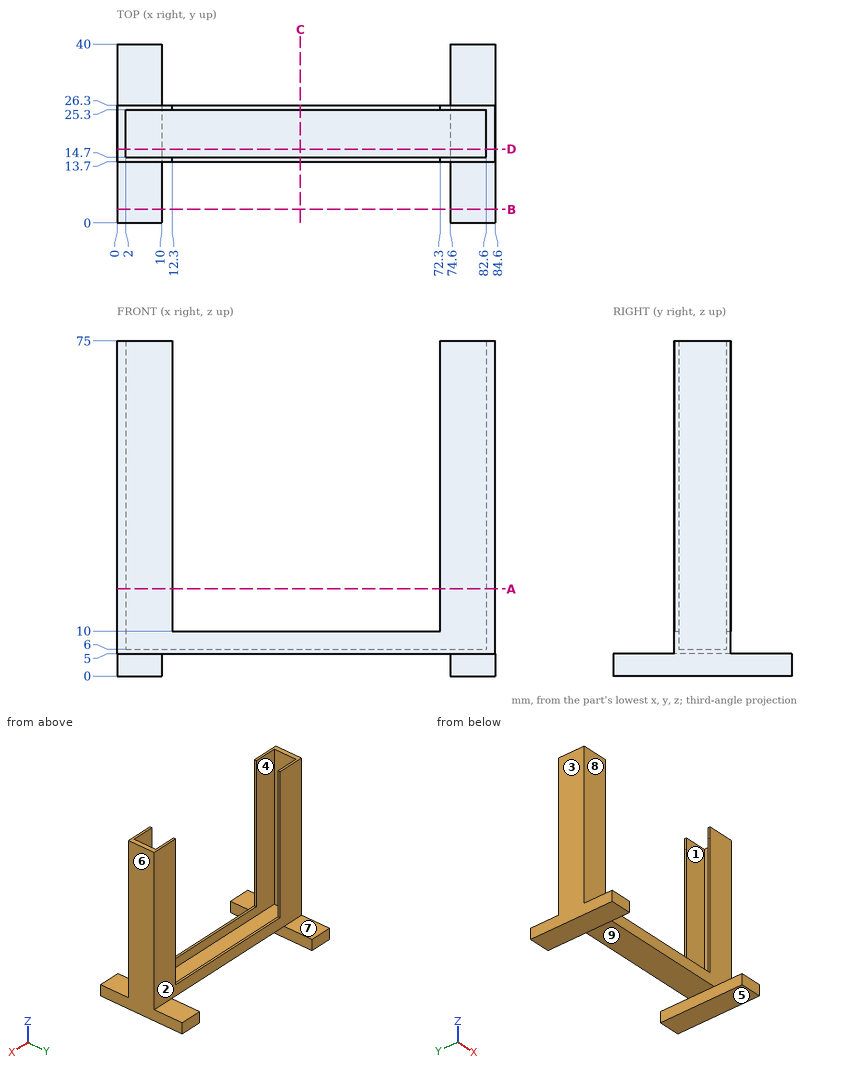
Could you check a few things on this drawing? It's one solid part, dimensions in mm from its lowest x, y, z. A direction names the side the tool comes from. Give positions to 0.01 mm unless a question says otherwise; leave off trailing zeros. Write each loop counter-clockwise with the first axis right and the second up, starting at its lowest first coordinate (ties: lowest second). Pieces come first, ordered by that corner, then holes. Notation, with made-up numbers: M -2.75,85 L 38.25,85 A8 cw 38.25,91 Z; hole C 8.25,-17 d8. An arc over 180 degrees is marked long. Put each result on its own line as item: value. Start each with the question number.
Item 1: Will these pins go through, and if not, where does the flat tip stop? pin 1 (5 mm diameter, centred on x = 3.5, y = 31.5, fed in from +Z); pin 2 (8.5 mm diameter, centred on x = 41.5, y = 22.5, fed in from +Z); pin 3 (6.5 mm diameter, centred on x = 37.5, y = 23, fed in from -Z).
Item 2: If we section it at B-B, the plane y = 3: Write out the boundary of the cut face in (x, z), then the cut area to 3 significant figures.
Item 3: Thinking about a two-plate mould opening in Y: for the marked faces 1, 2, 3 and 4, which applies, +Y half, -Y half, draft (parallel to the pull), parting line (faces both ways), or undercut?
Item 4: If we section it at C-C, the plane x = 41: Write out the boundary of the cut face in (y, z), then the cut area to 3 significant figures.
Item 5: If we section it at A-A, the plane z = 19.5: Write out the boundary of the cut face in (x, y), then the cut area to 3 significant figures.
Item 6: If we section it at D-D, the plane y = 16.5: Write out the boundary of the cut face in (x, z).
Item 7: On a 3-axis mill with a long thin cutter (end or side, diameter ignored), from which of +Z, -Z, +X, -X, +Y, -Y can I reach the whole of each face in a straight line? I mean the marked faces 5, 6, 7, 8 and 9. Say none if no direction works.
Item 8: I need wall thicknesses on L1, parallel to Y at x = 80, z = 41.5; L2, parallel to X at y = 16, z = 17; L3, parallel to X at y = 25.5, z = 63.5. Which ranges of each line are inside material? Lowest first, please. Write a range as from..to.
Values:
1. pin 1: z = 5
1. pin 2: z = 10
1. pin 3: z = 5
2. outline: M 0,0 L 10,0 L 10,5 L 0,5 Z; M 74.6,0 L 84.6,0 L 84.6,5 L 74.6,5 Z
2. area: 100 mm²
3. face 1: undercut
3. face 2: +Y half
3. face 3: draft
3. face 4: undercut
4. outline: M 13.7,5 L 26.3,5 L 26.3,10 L 25.3,10 L 25.3,6 L 14.7,6 L 14.7,10 L 13.7,10 Z
4. area: 20.6 mm²
5. outline: M 0,13.7 L 12.3,13.7 L 12.3,14.7 L 2,14.7 L 2,25.3 L 12.3,25.3 L 12.3,26.3 L 0,26.3 Z; M 72.3,13.7 L 84.6,13.7 L 84.6,26.3 L 72.3,26.3 L 72.3,25.3 L 82.6,25.3 L 82.6,14.7 L 72.3,14.7 Z
5. area: 91.6 mm²
6. outline: M 0,0 L 10,0 L 10,5 L 74.6,5 L 74.6,0 L 84.6,0 L 84.6,75 L 82.6,75 L 82.6,6 L 2,6 L 2,75 L 0,75 Z
7. face 5: -Z, +X, -X, +Y, -Y
7. face 6: +Z, -Z, +X, +Y, -Y
7. face 7: +Z, +X, -X, +Y
7. face 8: +Z, +X, -X, -Y
7. face 9: -Z, +Y, -Y
8. L1: 13.7..14.7, 25.3..26.3
8. L2: 0..2, 82.6..84.6
8. L3: 0..12.3, 72.3..84.6
